Could you check a few things on this model? Use its own coordinates, in mm. A direction names the side the tool comes from. Give positions to 0.01 mm unless a question says otherwise; leave off trailing zeros. Order: outer loops, then holes, each group sorted by start corner. A loop starts at its lowest first (then second) coordinate and runs counter-clockwise, first axis right, second up.
from build123d import *

# Parameters (mm, degrees)
F1_DEPTH = 6.985


with BuildPart() as f1:
    # F0 (on Top) → F1 (new body)
    with BuildSketch(Plane.XY):
        with BuildLine():
            Line((0, 18.1991), (0, 16.0909))
            ThreePointArc((0, 16.0909), (7.068545098, 14.4551974392), (12.7, 9.8806408097))
            ThreePointArc((12.7, 9.8806408097), (14.9827505764, 17.145), (12.7, 24.4093591903))
            ThreePointArc((12.7, 24.4093591903), (7.068545098, 19.8348025608), (0, 18.1991))
        make_face()
        with BuildLine():
            ThreePointArc((-12.7, 9.8806408097), (-7.068545098, 14.4551974392), (0, 16.0909))
            Line((0, 16.0909), (0, 18.1991))
            ThreePointArc((0, 18.1991), (-7.068545098, 19.8348025608), (-12.7, 24.4093591903))
            ThreePointArc((-12.7, 24.4093591903), (-14.9827505764, 17.145), (-12.7, 9.8806408097))
        make_face()
        with BuildLine():
            Line((0, -18.1991), (0, -16.0909))
            ThreePointArc((0, -16.0909), (-7.068545098, -14.4551974392), (-12.7, -9.8806408097))
            ThreePointArc((-12.7, -9.8806408097), (-14.9827505764, -17.145), (-12.7, -24.4093591903))
            ThreePointArc((-12.7, -24.4093591903), (-7.068545098, -19.8348025608), (0, -18.1991))
        make_face()
        with BuildLine():
            ThreePointArc((12.7, -9.8806408097), (7.068545098, -14.4551974392), (0, -16.0909))
            Line((0, -16.0909), (0, -18.1991))
            ThreePointArc((0, -18.1991), (7.068545098, -19.8348025608), (12.7, -24.4093591903))
            ThreePointArc((12.7, -24.4093591903), (14.9827505764, -17.145), (12.7, -9.8806408097))
        make_face()
        with BuildLine():
            ThreePointArc((0, -11.0109), (-11.0109, 0), (0, 11.0109))
            Line((0, 11.0109), (0, 16.0909))
            ThreePointArc((0, 16.0909), (-7.068545098, 14.4551974392), (-12.7, 9.8806408097))
            ThreePointArc((-12.7, 9.8806408097), (-16.0909, 0), (-12.7, -9.8806408097))
            ThreePointArc((-12.7, -9.8806408097), (-7.068545098, -14.4551974392), (0, -16.0909))
            Line((0, -16.0909), (0, -11.0109))
        make_face()
        with BuildLine():
            ThreePointArc((0, 11.0109), (7.785882057, 7.785882057), (11.0109, 0))
            ThreePointArc((11.0109, 0), (7.785882057, -7.785882057), (0, -11.0109))
            Line((0, -11.0109), (0, -16.0909))
            ThreePointArc((0, -16.0909), (7.068545098, -14.4551974392), (12.7, -9.8806408097))
            ThreePointArc((12.7, -9.8806408097), (15.2195843046, -5.2231519607), (16.0909, 0))
            ThreePointArc((16.0909, 0), (15.2195843046, 5.2231519607), (12.7, 9.8806408097))
            ThreePointArc((12.7, 9.8806408097), (7.068545098, 14.4551974392), (0, 16.0909))
            Line((0, 16.0909), (0, 11.0109))
        make_face()
        with BuildLine():
            Line((-13.5509, 34.29), (-11.0109, 34.29))
            ThreePointArc((-11.0109, 34.29), (0, 45.3009), (11.0109, 34.29))
            Line((11.0109, 34.29), (13.5509, 34.29))
            ThreePointArc((13.5509, 34.29), (14.2253166004, 36.013716502), (15.8904264404, 36.8220762927))
            ThreePointArc((15.8904264404, 36.8220762927), (0, 50.3809), (-15.8904264404, 36.8220762927))
            ThreePointArc((-15.8904264404, 36.8220762927), (-14.2253166004, 36.013716502), (-13.5509, 34.29))
        make_face()
        with BuildLine():
            ThreePointArc((-12.7, 24.4093591903), (-7.068545098, 19.8348025608), (0, 18.1991))
            Line((0, 18.1991), (0, 23.2791))
            ThreePointArc((0, 23.2791), (-7.785882057, 26.504117943), (-11.0109, 34.29))
            Line((-11.0109, 34.29), (-13.5509, 34.29))
            ThreePointArc((-13.5509, 34.29), (-14.2253166004, 32.566283498), (-15.8904264404, 31.7579237073))
            ThreePointArc((-15.8904264404, 31.7579237073), (-14.7598601323, 27.8819120103), (-12.7, 24.4093591903))
        make_face()
        with BuildLine():
            Line((0, 23.2791), (0, 18.1991))
            ThreePointArc((0, 18.1991), (7.068545098, 19.8348025608), (12.7, 24.4093591903))
            ThreePointArc((12.7, 24.4093591903), (14.7598601323, 27.8819120103), (15.8904264404, 31.7579237073))
            ThreePointArc((15.8904264404, 31.7579237073), (14.2253166004, 32.566283498), (13.5509, 34.29))
            Line((13.5509, 34.29), (11.0109, 34.29))
            ThreePointArc((11.0109, 34.29), (7.785882057, 26.504117943), (0, 23.2791))
        make_face()
        with BuildLine():
            ThreePointArc((12.7, -24.4093591903), (7.068545098, -19.8348025608), (0, -18.1991))
            Line((0, -18.1991), (0, -23.2791))
            ThreePointArc((0, -23.2791), (7.785882057, -26.504117943), (11.0109, -34.29))
            Line((11.0109, -34.29), (13.5509, -34.29))
            ThreePointArc((13.5509, -34.29), (14.2253166004, -32.566283498), (15.8904264404, -31.7579237073))
            ThreePointArc((15.8904264404, -31.7579237073), (14.7598601323, -27.8819120103), (12.7, -24.4093591903))
        make_face()
        with BuildLine():
            Line((0, -23.2791), (0, -18.1991))
            ThreePointArc((0, -18.1991), (-7.068545098, -19.8348025608), (-12.7, -24.4093591903))
            ThreePointArc((-12.7, -24.4093591903), (-14.7598601323, -27.8819120103), (-15.8904264404, -31.7579237073))
            ThreePointArc((-15.8904264404, -31.7579237073), (-14.2253166004, -32.566283498), (-13.5509, -34.29))
            Line((-13.5509, -34.29), (-11.0109, -34.29))
            ThreePointArc((-11.0109, -34.29), (-7.785882057, -26.504117943), (0, -23.2791))
        make_face()
        with BuildLine():
            Line((13.5509, -34.29), (11.0109, -34.29))
            ThreePointArc((11.0109, -34.29), (0, -45.3009), (-11.0109, -34.29))
            Line((-11.0109, -34.29), (-13.5509, -34.29))
            ThreePointArc((-13.5509, -34.29), (-14.2253166004, -36.013716502), (-15.8904264404, -36.8220762927))
            ThreePointArc((-15.8904264404, -36.8220762927), (0, -50.3809), (15.8904264404, -36.8220762927))
            ThreePointArc((15.8904264404, -36.8220762927), (14.2253166004, -36.013716502), (13.5509, -34.29))
        make_face()
    extrude(amount=F1_DEPTH)


solid = f1.part
Item 1: For pin 1 (1.5 mm diameter, centred on x = 8, z = 4, fed in from +Y), with a flat end and sliding along its axis, tell me the tip position at first contact or that it passes through.
Findings:
pin 1: stops at y = 48.66
Item 2: Imagine slicing it at C-C on y = -26. List the corners of the cut face in (x, z) for me (3 decimals), then the cut area to 3 significant figures.
Findings:
outline: (-13.791, 0) - (-7.247, 0) - (-7.247, 6.985) - (-13.791, 6.985) - close; (7.247, 0) - (13.791, 0) - (13.791, 6.985) - (7.247, 6.985) - close
area: 91.4 mm2
Item 3: Imagine slicing it at A-A on x = 2.5. List the corners of the cut face in (y, z) for me (1 decimal).
Findings:
outline: (-50.2, 0) - (-45, 0) - (-45, 7) - (-50.2, 7) - close; (-23.6, 0) - (-10.7, 0) - (-10.7, 7) - (-23.6, 7) - close; (10.7, 0) - (23.6, 0) - (23.6, 7) - (10.7, 7) - close; (45, 0) - (50.2, 0) - (50.2, 7) - (45, 7) - close
Item 4: Imagine slicing it at B-B on z = 3.75. List the corners of the cut face in (x, y) for me (3 decimals).
Findings:
outline: (-15.89, -36.822) arc R16.091 ccw to (15.89, -36.822) arc R2.54 cw to (15.89, -31.758) arc R16.091 ccw to (12.7, -24.409) arc R12.7 ccw to (12.7, -9.881) arc R16.091 ccw to (12.7, 9.881) arc R12.7 ccw to (12.7, 24.409) arc R16.091 ccw to (15.89, 31.758) arc R2.54 cw to (15.89, 36.822) arc R16.091 ccw to (-15.89, 36.822) arc R2.54 cw to (-15.89, 31.758) arc R16.091 ccw to (-12.7, 24.409) arc R12.7 ccw to (-12.7, 9.881) arc R16.091 ccw to (-12.7, -9.881) arc R12.7 ccw to (-12.7, -24.409) arc R16.091 ccw to (-15.89, -31.758) arc R2.54 cw to start; hole circle Ø22.022 at (0, -34.29); hole circle Ø22.022 at (0, 0); hole circle Ø22.022 at (0, 34.29)
Item 5: We'd pull the mould along Y, two halves only. Please class faces 4 (the cylindrical face through (0.318, 50.378, 3.444)), 5 (the cylindrical face through (-0.318, -50.378, 3.444)), 6 (the flat face through (0, 12, 6.985)), 7 (the cylindrical face through (14.78, -27.93, 3.44)): +Y half, -Y half, draft (parallel to the pull), parting line (faces both ways), or undercut.
Findings:
face 4: +Y half
face 5: -Y half
face 6: draft
face 7: undercut
Item 6: Please list where these lines run through material, in increasing order: line 1 along Y through (x, z) = (9, 0.5); line 2 along Y through (x, z) = (-13, 6.5); line 3 along Y through (x, z) = (-6.5, 4.75).
Findings:
line 1: y = -47.63 to -40.63, -27.95 to -6.34, 6.34 to 27.95, 40.63 to 47.63
line 2: y = -43.77 to -24.81, -23.96 to -10.33, -9.48 to 9.48, 10.33 to 23.96, 24.81 to 43.77
line 3: y = -49.01 to -43.18, -25.4 to -8.89, 8.89 to 25.4, 43.18 to 49.01
Item 7: For faces 1 (the cylindrical face through (-14.737, -27.83, 3.444)), 2 (the flat face through (0, 12, 0)), 3 (the cylindrical face through (14.737, 27.83, 3.444)), which set-ups out of +Z, -Z, +X, -X, +Y, -Y let a thin tool reach every point of the face, with its end or its side?
Findings:
face 1: +Z, -Z, -X
face 2: -Z, +X, -X, +Y, -Y
face 3: +Z, -Z, +X
Item 8: Imagine slicing it at D-D on x = 9. List the corners of the cut face in (y, z) for me (1 decimal), then the cut area to 3 significant figures.
Findings:
outline: (-47.6, 0) - (-40.6, 0) - (-40.6, 7) - (-47.6, 7) - close; (-27.9, 0) - (-6.3, 0) - (-6.3, 7) - (-27.9, 7) - close; (6.3, 0) - (27.9, 0) - (27.9, 7) - (6.3, 7) - close; (40.6, 0) - (47.6, 0) - (47.6, 7) - (40.6, 7) - close
area: 400 mm2
